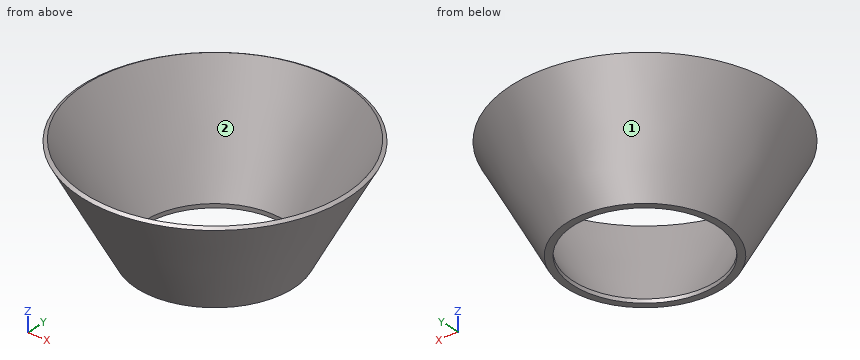
```python
from build123d import *

# Parameters (mm, degrees)
SKETCH_1_R          = 100
SKETCH_1_R_2        = 95
EXTRUDE_1_DEPTH     = 70
EXTRUDE_START       = 5
SKETCH_2_R          = 100
EXTRUDE_2_DEPTH     = 5
SKETCH_6_R          = 100
CUT_EXTRUDE_1_DEPTH = 75
EXTRUDE_3_REACH     = 223.205
SKETCH_8_R          = 80
SKETCH_8_R_2        = 73.07179677


with BuildPart() as part:
    # 草图1 → 凸台-拉伸1 (new body)
    with BuildSketch(Plane.XY):
        Circle(SKETCH_1_R)
        Circle(SKETCH_1_R_2, mode=Mode.SUBTRACT)
    extrude(amount=EXTRUDE_1_DEPTH)

    # 草图2 → 凸台-拉伸2 (add)
    with BuildSketch(Plane(origin=(0, 0, 0), x_dir=(-1, 0, 0), z_dir=(0, 0, -1)).offset(EXTRUDE_START)):
        Circle(SKETCH_2_R)
    extrude(amount=-EXTRUDE_2_DEPTH)

    # 草图6 → 切除-拉伸1 (cut)
    with BuildSketch(Plane(origin=(0, 0, -5), x_dir=(-1, 0, 0), z_dir=(0, 0, -1))):
        Circle(SKETCH_6_R)
    extrude(amount=-CUT_EXTRUDE_1_DEPTH, mode=Mode.SUBTRACT)


with BuildPart() as body_2:
    # 草图5 → 旋转1 (revolve)
    with BuildSketch(Plane(origin=(0, 0, 0), x_dir=(0, 0, -1), z_dir=(1, 0, 0))):
        Polygon((-75.339745962, 73.07179677), (-71.339745962, 80), (-177.262794416, 136.535898385), (-179.262794416, 133.07179677), align=None)
    revolve(axis=Axis((0, 0, 0), (0, 0, 1)))

    # 凸台-拉伸3: up to this cone (the profile starts outside it)
    extrude_3_end = Plane(origin=(0, 0, 71.339746), z_dir=(0, 0, 1)).offset(-122.564063643) * Cone(1e-06, 240.773225898, 417.031459358, align=(Align.CENTER, Align.CENTER, Align.MIN), mode=Mode.PRIVATE)
    # 草图8 → 凸台-拉伸3 (add, up to the surface)
    with BuildSketch(Plane(origin=(0, 0, 71.339745962), x_dir=(-1, 0, 0), z_dir=(0, 0, -1)), mode=Mode.PRIVATE) as extrude_3_sk1:
        Circle(SKETCH_8_R)
        with Locations(Location((0, 0, 0), (0, 0, 90))):
            Circle(SKETCH_8_R_2, mode=Mode.SUBTRACT)
    extrude_3_tool1 = extrude(extrude_3_sk1.sketch, amount=-EXTRUDE_3_REACH, mode=Mode.PRIVATE) - extrude_3_end
    add(extrude_3_tool1.solids().sort_by_distance((77.737258, 0, 71.339746))[0])


solid = body_2.part
```
The listing builds one solid part. Answer for the finished solid, in the listing's coordinates (mm). Face numbers are marked on the shaded views. Give positions to 0.01 mm unless a question says otherwise; leave off trailing zeros. Loops run counter-clockwise (first coordinate to the right, second up) from the corner with the lowest first, then second, coordinate; pieces in that order, holes last. Notation, with made-up numbers: (35.25, 66.25) - (64.25, 66.25) arc R15 ccw to (64.25, 89.25) - close; hole circle Ø3 at (64, 54.25). An arc over 180 degrees is marked (long way). Answer as CSV lines item,"result". Start each with the question number.
Item 1: A cutting plane is placed at A-A on y = 0. Determine the outline of the cut face in (x, z), then the cut area to 3 significant figures.
Item 2: Find the intervals of material crossed by line 1 (X direction, y = 0, z = 72.3); line 2 (Y direction, x = -41.5, z = 116.5); line 3 (X direction, y = -53, z = 88), in increasing order. Write a range as from..to.
Item 3: A cutting plane is placed at D-D on z = 157.5. Determine the outline of the cut face in (x, y).
Item 4: A cutting plane is placed at C-C on z = 86. Determine the outline of the cut face in (x, y).
Item 5: The mould has two halves that part along X. Classify the marked faces 1 and 2: +X half, -X half, draft (parallel to the pull), parting line (faces both ways), or undercut.
Item 6: Each of these flat-tipped pins is pushed along its axis until it touches: pin 1 (2 mm diameter, centred on x = 43, z = 145, fed in from -Y); pin 2 (8 mm diameter, centred on y = -31, z = 150, fed in from +X); pin 3 (1.5 mm diameter, centred on y = 18.5, z = 125, fed in from -X); pin 4 (12 mm diameter, centred on x = -97.5, z = 89, fed in from -Y). Where does it stop, or does it pass through?
Found:
1,outline,"(-136.54, 177.26) - (-80, 71.34) - (-73.07, 71.34) - (-73.07, 75.34) - (-133.07, 179.26) - close; (73.07, 71.34) - (80, 71.34) - (136.54, 177.26) - (133.07, 179.26) - (73.07, 75.34) - close"
1,area,"1,470 mm^2"
2,line 1,"x = -80.51..-73.07, 73.07..80.51"
2,line 2,"y = -95.47..-87.49, 87.49..95.47"
2,line 3,"x = -71.36..-60.43, 60.43..71.36"
3,outline,"circle Ø251.98 at (0, 0); hole circle Ø241.01 at (0, 0)"
4,outline,"circle Ø175.65 at (0, 0); hole circle Ø158.45 at (0, 0)"
5,face 1,"parting line"
5,face 2,"undercut"
6,pin 1,"stops at y = -111.99"
6,pin 2,"stops at x = 120.4"
6,pin 3,"stops at x = -107.48"
6,pin 4,"passes through"
